Could you check a few things on this model? Use its own coordinates, in mm. A direction names the side the tool comes from. Give positions to 0.01 mm unless a question says otherwise; leave off trailing zeros. Loops run counter-clockwise (first coordinate to the right, second up) from the corner with the lowest first, then second, coordinate; pieces in that order, holes last. Notation, with made-up numbers: (18.5, -25) -> (29.5, -25) arc R26 ccw to (29.5, 13) -> close; hole circle Ø4 at (-21.75, 30). An arc over 180 degrees is marked (long way). Put each result on its own line as item: value.
```python
from build123d import *

# Parameters (mm, degrees)
EXTRUDE_1_DEPTH = 2.1
SKETCH_2_R      = 6
EXTRUDE_2_DEPTH = 13.2
SKETCH_3_R      = 4
SKETCH_3_W      = 2
SKETCH_3_H      = 12
EXTRUDE_3_DEPTH = 3


with BuildPart() as part:
    # Эскиз1 → Бобышка-Вытянуть1 (new body)
    with BuildSketch(Plane.XY):
        with BuildLine():
            Line((-94, 6), (94, 6))
            ThreePointArc((94, 6), (100, 0), (94, -6))
            Line((94, -6), (-94, -6))
            ThreePointArc((-94, -6), (-100, 0), (-94, 6))
        make_face()
    extrude(amount=EXTRUDE_1_DEPTH)

    # Эскиз2 → Бобышка-Вытянуть2 (add)
    with BuildSketch(Plane.XY.offset(2.1)):
        with Locations(Location((-94, 0, 0), (0, 0, 270))):
            Circle(SKETCH_2_R)
        with Locations(Location((94, 0, 0), (0, 0, 90))):
            Circle(SKETCH_2_R)
    extrude(amount=EXTRUDE_2_DEPTH)

    # Эскиз3 → Бобышка-Вытянуть3 (add)
    with BuildSketch(Plane.XY.offset(2.1)):
        with Locations((-72, 0)):
            Circle(SKETCH_3_R)
        with Locations((-36, 0)):
            Circle(SKETCH_3_R)
        Circle(SKETCH_3_R)
        with Locations((36, 0)):
            Circle(SKETCH_3_R)
        with Locations((72, 0)):
            Circle(SKETCH_3_R)
        with Locations((-54, 0)):
            Circle(SKETCH_3_R)
        with Locations((-18, 0)):
            Circle(SKETCH_3_R)
        with Locations((18, 0)):
            Circle(SKETCH_3_R)
        with Locations((54, 0)):
            Circle(SKETCH_3_R)
        with Locations((-81, 0)):
            Rectangle(SKETCH_3_W, SKETCH_3_H)
        with Locations((-63, 0)):
            Rectangle(SKETCH_3_W, SKETCH_3_H)
        with Locations((-45, 0)):
            Rectangle(SKETCH_3_W, SKETCH_3_H)
        with Locations((-27, 0)):
            Rectangle(SKETCH_3_W, SKETCH_3_H)
        with Locations((-9, 0)):
            Rectangle(SKETCH_3_W, SKETCH_3_H)
        with Locations((9, 0)):
            Rectangle(SKETCH_3_W, SKETCH_3_H)
        with Locations((27, 0)):
            Rectangle(SKETCH_3_W, SKETCH_3_H)
        with Locations((45, 0)):
            Rectangle(SKETCH_3_W, SKETCH_3_H)
        with Locations((63, 0)):
            Rectangle(SKETCH_3_W, SKETCH_3_H)
        with Locations((81, 0)):
            Rectangle(SKETCH_3_W, SKETCH_3_H)
    extrude(amount=EXTRUDE_3_DEPTH)


solid = part.part
```
1. I need wall thicknesses on line 1 (Z direction, x = 14, y = -1.75); line 2 (X direction, y = -5.5, z = 11); line 3 (X direction, y = 2, z = 9). Which ranges of each line are inside material? Lowest first, please.
Recorded:
line 1: z = 0 to 2.1
line 2: x = -96.4 to -91.6, 91.6 to 96.4
line 3: x = -99.66 to -88.34, 88.34 to 99.66
2. If we section it at A-A (x = -54): List the corners of the cut face in (y, z) for me, then the cut area to 3 significant figures.
Recorded:
outline: (-6, 0) -> (6, 0) -> (6, 2.1) -> (4, 2.1) -> (4, 5.1) -> (-4, 5.1) -> (-4, 2.1) -> (-6, 2.1) -> close
area: 49.2 mm^2
3. I'm going to push flat-ended pins straight in: pin 1 (2.5 mm diameter, centred on x = 37, y = -1, fed in from +Z); pin 2 (1.5 mm diameter, centred on y = 1, z = 3.5, fed in from -X); pin 3 (8 mm diameter, centred on x = 30.5, z = 6, fed in from +Y); pin 4 (6 mm diameter, centred on x = 59.5, z = 8.5, fed in from +Y). Where does each tip first touch, or does it pass through?
Recorded:
pin 1: stops at z = 5.1
pin 2: stops at x = -99.99
pin 3: stops at y = 6
pin 4: passes through
4. For faces 1 (the face through (-56, 4, 2.1)), 2 (the face through (-94, 0, 15.3)), 3 (the face through (36, 0, 5.1)), which set-ups out of +Z, -Z, +X, -X, +Y, -Y let a thin tool reach every point of the face, with its end or its side?
Recorded:
face 1: +Z
face 2: +Z, +X, -X, +Y, -Y
face 3: +Z, +Y, -Y
5. Thinking about a two-plate mould opening in X: for faces 4 (the face through (54, 0, 5.1)), 5 (the face through (94, 0, 15.3)), which applies, pulls with the +X half, pulls with the -X half, needs draft (parallel to the pull), parting line crosses it, or undercut?
Recorded:
face 4: undercut
face 5: needs draft
6. If we section it at B-B (z = 10.5): List the corners of the cut face in (x, y) for me, then the cut area to 3 significant figures.
Recorded:
outline: circle Ø12 at (-94, 0); circle Ø12 at (94, 0)
area: 226 mm^2
7. If we section it at C-C (x = 71.5): List the corners of the cut face in (y, z) for me.
Recorded:
outline: (-6, 0) -> (6, 0) -> (6, 2.1) -> (3.97, 2.1) -> (3.97, 5.1) -> (-3.97, 5.1) -> (-3.97, 2.1) -> (-6, 2.1) -> close
